Part print with two shaded views. Sizes in mm from the minimum x, y, z corner. Give positions to 0.01 mm unless a question says otherwise; leave off trailing zeros. Write each loop counter-clockwise with the first axis right and the second up, starting at its lowest first coordinate (ties: lowest second). Pieces come first, ordered by that corner, then holes. Notation, with made-up numbers: (-11.75, 84.25) -> (21.25, 84.25) arc R16 ccw to (21.25, 115.25) -> close; hole circle Ø7 at (88.5, 55). An arc over 180 degrees is marked (long way). Answer as a JSON object with one key per item and string values.
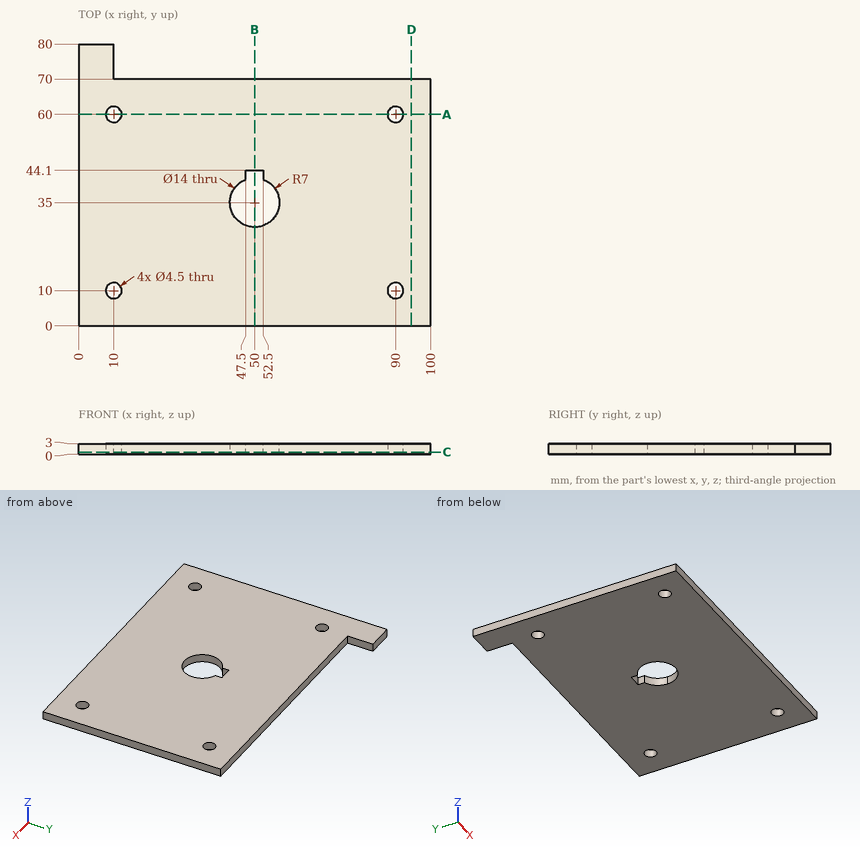
1) Wall check: probe 1 along X at (y, z) = (60, 0.8); probe 2 along Y at (x, z) = (90, 1.2); probe 3 along X at (y, z) = (35, 0.9). Give the ranges that are in metal, low to high.
Model answer:
{"probe 1": "x = 0 to 7.75, 12.25 to 87.75, 92.25 to 100", "probe 2": "y = 0 to 7.75, 12.25 to 57.75, 62.25 to 70", "probe 3": "x = 0 to 43, 57 to 100"}
2) Slice it at A-A (y = 60). List the corners of the cut face in (x, z).
Model answer:
{"outline": "(0, 0) -> (7.75, 0) -> (7.75, 3) -> (0, 3) -> close; (12.25, 0) -> (87.75, 0) -> (87.75, 3) -> (12.25, 3) -> close; (92.25, 0) -> (100, 0) -> (100, 3) -> (92.25, 3) -> close"}
3) Pin check, flat tips, straight feed: pin 1 (3.5 mm diameter, centred on x = 10, y = 60, fed in from +Z); pin 2 (6 mm diameter, centred on x = 90, y = 60, fed in from +Z); pin 3 (1.5 mm diameter, centred on y = 74, z = 1, fed in from +X). Stop position of each tip, or through.
Model answer:
{"pin 1": "passes through", "pin 2": "stops at z = 3", "pin 3": "stops at x = 10"}
4) Slice it at D-D (x = 94.5). List the corners of the cut face in (y, z), then the cut area to 3 significant figures.
Model answer:
{"outline": "(0, 0) -> (70, 0) -> (70, 3) -> (0, 3) -> close", "area": "210 mm2"}
5) Slice it at B-B (x = 50). List the corners of the cut face in (y, z), then the cut area to 3 significant figures.
Model answer:
{"outline": "(0, 0) -> (28, 0) -> (28, 3) -> (0, 3) -> close; (44.1, 0) -> (70, 0) -> (70, 3) -> (44.1, 3) -> close", "area": "162 mm2"}
6) Slice it at C-C (z = 0.65). List the corners of the cut face in (x, y), then the cut area to 3 significant figures.
Model answer:
{"outline": "(0, 0) -> (100, 0) -> (100, 70) -> (10, 70) -> (10, 80) -> (0, 80) -> close; hole circle Ø4.5 at (10, 10); hole circle Ø4.5 at (10, 60); hole (47.5, 41.54) arc R7 ccw (long way) to (52.5, 41.54) -> (52.5, 44.1) -> (47.5, 44.1) -> close; hole circle Ø4.5 at (90, 10); hole circle Ø4.5 at (90, 60)", "area": "6,870 mm2"}
